from build123d import *

# Parameters (mm, degrees)
SKETCH1_R           = 5.08
SKETCH1_R_2         = 1.75
BOSS_EXTRUDE1_DEPTH = 6.35
CUT_EXTRUDE1_DEPTH  = 7.35
CIRPATTERN1_COUNT   = 2
CIRPATTERN1_ANGLE   = 60


with BuildPart() as part:
    # Sketch1 → Boss-Extrude1 (new body)
    with BuildSketch(Plane(origin=(0, 0, 0), x_dir=(1, 0, 0), z_dir=(0, 1, 0))):
        with BuildLine():
            Line((-17.104001725, 6.625), (-2.814582562, -18.125))
            ThreePointArc((-2.814582562, -18.125), (0, -19.75), (2.814582562, -18.125))
            Line((2.814582562, -18.125), (17.104001725, 6.625))
            ThreePointArc((17.104001725, 6.625), (17.539419162, 8.25), (17.104001725, 9.875))
            ThreePointArc((17.104001725, 9.875), (0, 19.75), (-17.104001725, 9.875))
            ThreePointArc((-17.104001725, 9.875), (-17.539419162, 8.25), (-17.104001725, 6.625))
        make_face()
        Circle(SKETCH1_R, mode=Mode.SUBTRACT)
        with Locations((-14.289419162, 8.25)):
            Circle(SKETCH1_R_2, mode=Mode.SUBTRACT)
        with Locations((0, -16.5)):
            Circle(SKETCH1_R_2, mode=Mode.SUBTRACT)
        with Locations((14.289419162, 8.25)):
            Circle(SKETCH1_R_2, mode=Mode.SUBTRACT)
    extrude(amount=BOSS_EXTRUDE1_DEPTH)

    # Sketch2 → Cut-Extrude1 (cut, through all)
    with BuildSketch(Plane(origin=(0, 6.35, 0), x_dir=(1, 0, 0), z_dir=(0, 1, 0))):
        with BuildLine():
            ThreePointArc((8.036161973, 16.182379357), (7.2975, 12.639640768), (9.99627063, 15.050710096))
            ThreePointArc((9.99627063, 15.050710096), (10.255103275, 16.120005739), (11.354562521, 16.159715652))
            ThreePointArc((11.354562521, 16.159715652), (9.875, 17.104001725), (8.317443012, 17.913197418))
            ThreePointArc((8.317443012, 17.913197418), (8.832782842, 16.941182824), (8.036161973, 16.182379357))
        make_face()
    cut_extrude1 = extrude(amount=-CUT_EXTRUDE1_DEPTH, mode=Mode.SUBTRACT)

    # CirPattern1: Cut-Extrude1 ×2 about axis
    cirpattern1_axis = Axis((0, 0, 0), (0, 1, 0))
    for i in range(1, CIRPATTERN1_COUNT):
        add(cut_extrude1.rotate(cirpattern1_axis, i * CIRPATTERN1_ANGLE / (CIRPATTERN1_COUNT - 1)), mode=Mode.SUBTRACT)


solid = part.part
Work out the finished part from the listing and answer in its coordinate system (mm). A direction names the side the tool comes from. Round coordinates to 2 decimals unless told otherwise and drop trailing zeros. Loops run counter-clockwise (first coordinate to the right, second up) from the corner with the lowest first, then second, coordinate; pieces in that order, holes last. Notation, with made-up numbers: M 81,58.25 L 109,58.25 A22 cw 109,73.25 Z; hole C 14,29 d5. An arc over 180 degrees is marked long. One line per question, with ' | ' between items. Start each with the question number.
(1) A cutting plane is placed at B-B on x = -7. Write down the section's boundary in (y, z).
(2) Find the intervals of material crossed by line 1 (Z direction, x = 0, y = 1.5); line 2 (X direction, y = 3.25, z = -8.25); line 3 (Z direction, x = -1, y = 2.5), in increasing order.
(3) A tool of negligible diameter and unlimited length cuts with its end or side. For faces 4 (the face through (-8.83, 3.22, -16.92)), 5 (the face through (-4, 6.35, -5)), from which of +Z, -Z, +X, -X, +Y, -Y can it reach the whole face along a straight path? Write none if from no direction.
(4) A cutting plane is placed at D-D on x = 0. Write down the section's boundary in (y, z).
(5) For a pull along X with two mould halves and no side action, classify faces 1 (the face through (-0.05, 3.13, 19.75)), 2 (the face through (-14.531, 3.131, -13.375)), 3 (the face through (-10.27, 3.22, -16.13)) as released by +X, released by -X, zero draft, split by the parting line, or undercut.
(6) Flat-ended cylindrical pins translate along their axes: pin 1 Ø3 at (x, y) = (-12, 4.5) entering from +Z; pin 2 Ø4.5 at (x, z) = (-14.29, -8.25) entering from +Y; pin 3 Ø3 at (x, y) = (-4, 3.5) entering from -Z; pin 4 Ø2 at (x, z) = (0, 16.5) entering from -Y. Find the tip coordinate at first contact, or state that the pin passes through.
(7) A cutting plane is placed at A-A on z = -8.25. Write down the section's boundary in (x, y), plus the area to 3 significant figures.
(8) A cutting plane is placed at C-C on z = 0. Write down the section's boundary in (x, y).
Geometry check:
1) outline: M 0,-18.47 L 6.35,-18.47 L 6.35,-15.73 L 0,-15.73 Z; M 0,-12.85 L 6.35,-12.85 L 6.35,10.88 L 0,10.88 Z
2) line 1: z = -19.75 to -5.08, 5.08 to 14.75, 18.25 to 19.75 | line 2: x = -17.54 to -16.04, -12.54 to 12.54, 16.04 to 17.54 | line 3: z = -19.72 to -4.98, 4.98 to 15.06, 17.94 to 19.59
3) face 4: +Y, -Y | face 5: +Z, -Z, +X, -X, +Y
4) outline: M 0,-19.75 L 6.35,-19.75 L 6.35,-5.08 L 0,-5.08 Z; M 0,5.08 L 6.35,5.08 L 6.35,14.75 L 0,14.75 Z; M 0,18.25 L 6.35,18.25 L 6.35,19.75 L 0,19.75 Z
5) face 1: split by the parting line | face 2: released by -X | face 3: undercut
6) pin 1: stops at z = 4.81 | pin 2: stops at y = 6.35 | pin 3: stops at z = -19.59 | pin 4: passes through
7) outline: M -17.54,0 L -16.04,0 L -16.04,6.35 L -17.54,6.35 Z; M -12.54,0 L 12.54,0 L 12.54,6.35 L -12.54,6.35 Z; M 16.04,0 L 17.54,0 L 17.54,6.35 L 16.04,6.35 Z | area: 178 mm²
8) outline: M -13.28,0 L -5.08,0 L -5.08,6.35 L -13.28,6.35 Z; M 5.08,0 L 13.28,0 L 13.28,6.35 L 5.08,6.35 Z
